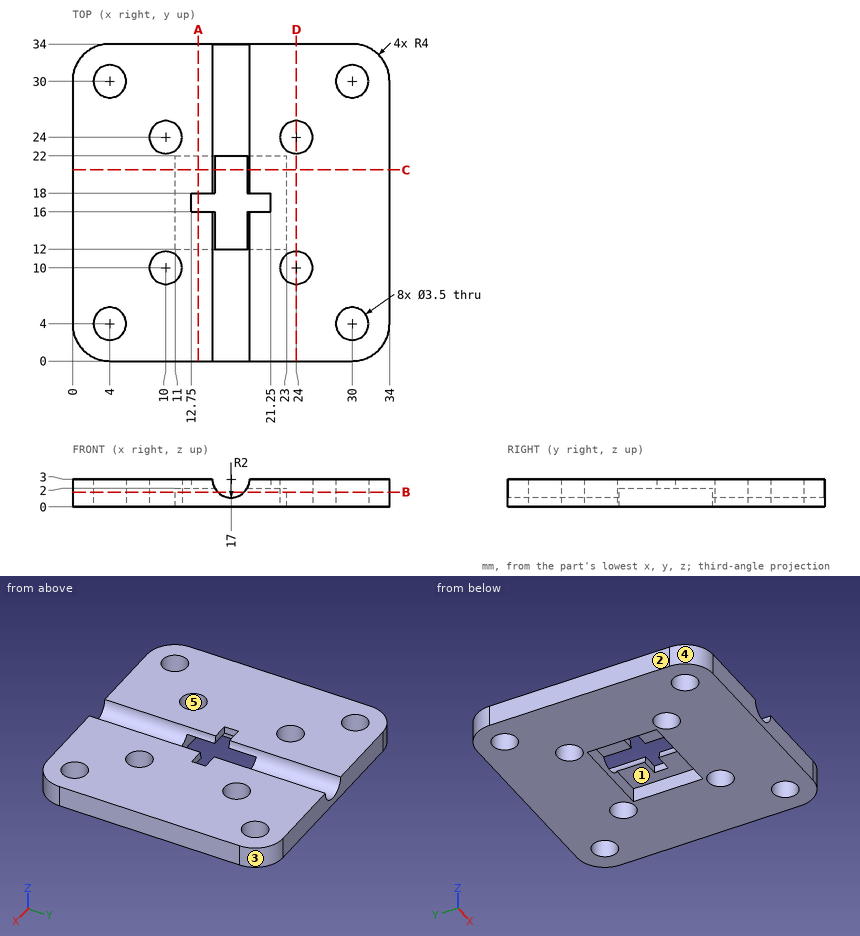
Part print with two shaded views. Sizes in mm from the minimum x, y, z corner. A direction names the side the tool comes from. Give positions to 0.01 mm unless a question says otherwise; leave off trailing zeros. Write each loop counter-clockwise with the first axis right and the second up, starting at its lowest first coordinate (ties: lowest second). Pieces come first, ordered by that corner, then holes.
1) Pin check, flat tips, straight feed: pin 1 (3 mm diameter, centred on x = 24, y = 24, fed in from -Z); pin 2 (1.3 mm diameter, centred on x = 13.5, y = 14.5, fed in from -Z). Stop position of each tip, or through.
Resolved:
pin 1: passes through
pin 2: stops at z = 2
2) Probe L1, parallel to Y at x = 10, z = 1.1; L2, parallel to Y at x = 30, z = 1.45; L3, parallel to Y at x = 15.5, z = 0.55. List the from-to ranges inside material, lowest first.
Resolved:
L1: y = 0 to 8.25, 11.75 to 22.25, 25.75 to 34
L2: y = 0 to 2.25, 5.75 to 28.25, 31.75 to 34
L3: y = 0 to 12, 22 to 34
3) Cut at D-D on x = 24. Write the cut outline in (y, z).
Resolved:
outline: (0, 0) - (8.25, 0) - (8.25, 3) - (0, 3) - close; (11.75, 0) - (22.25, 0) - (22.25, 3) - (11.75, 3) - close; (25.75, 0) - (34, 0) - (34, 3) - (25.75, 3) - close
4) Cut at C-C on y = 20.5. Write the cut outline in (x, z).
Resolved:
outline: (0, 0) - (11, 0) - (11, 2) - (15.27, 2) arc R2 cw to (15, 3) - (0, 3) - close; (18.73, 2) - (23, 2) - (23, 0) - (34, 0) - (34, 3) - (19, 3) arc R2 cw to start
5) Two-plate mould, pull along X, no slides. Class the marked faces 3, 4 and 5: released by +X, released by -X, zero draft, split by the parting line, or undercut.
Resolved:
face 3: released by +X
face 4: released by -X
face 5: undercut
6) Which spindle directions (+Z, -Z, +X, -X, +Y, -Y) get a long thin tool onto all of the face, cutting with end or side? Do the marked faces 1 and 2. Say none if no direction does.
Resolved:
face 1: -Z
face 2: +Z, -Z, -X, +Y, -Y
7) Cut at A-A on x = 13.5. Write the cut outline in (y, z).
Resolved:
outline: (0, 0) - (12, 0) - (12, 2) - (16, 2) - (16, 3) - (0, 3) - close; (18, 2) - (22, 2) - (22, 0) - (34, 0) - (34, 3) - (18, 3) - close
8) Cut at B-B on z = 1.6. State how many separate pieces and enclosed holes the cut face has, then the cut area to 3 significant figures.
Resolved:
separate pieces: 2
enclosed holes: 8
area: 877 mm2
